Autodesk Inventor part; units mm, degrees
ref_plane "YZ Plane" through (0, 0, 0) normal (1, 0, 0) x (0, 1, 0)
ref_plane "XZ Plane" through (0, 0, 0) normal (0, 1, 0) x (-1, 0, 0)
ref_plane "XY Plane" through (0, 0, 0) normal (0, 0, 1) x (1, 0, 0)
sketch "Sketch1" plane through (0, 0, 0) normal (0, 0, 1) x (1, 0, 0)
  line L0 (0, 4) -> (0, 0)
  line L1 (0, 0) -> (125, 0)
  line L2 (125, 0) -> (125, 23.5)
  line L3 (57, 23.5) -> (0, 4)
  line L4 (81, 23.5) -> (81, 14.5)
  line L5 (81, 14.5) -> (92, 14.5)
  line L6 (92, 14.5) -> (92, 23.5)
  line L7 (125, 23.5) -> (92, 23.5)
  line L8 (81, 23.5) -> (57, 23.5)
  circle A0 centre (99.5, 19) radius 2.25
  circle A1 centre (119.5, 19) radius 2.25
  circle A2 centre (28.2, 6) radius 2.25
  circle A3 centre (28.2, 6) radius 4.5 construction
  point P0 (92, 19)
  dimension "d0" = 4
  dimension "d1" = 125
  dimension "d2" = 9
  dimension "d3" = 11
  dimension "d4" = 33
  dimension "d5" = 24
  dimension "d6" = 23.5
  dimension "d7" = 4.5
  dimension "d8" = 4.5
  dimension "d9" = 5.5
  dimension "d10" = 20
  dimension "d11" = 4.5
  dimension "d12" = 9
  dimension "d13" = 6
  dimension "d14" = 28.2
extrude "Extrusion1" add sketch "Sketch1" along normal blind 6.5
sketch "Sketch2" plane through (0, 0, 6.5) normal (0, 0, 1) x (1, 0, 0)
  line L0 (0, 0) -> (125, 0)
  line L1 (125, 23.5) -> (92, 23.5)
  line L2 (17, 0) -> (25, 0)
  line L3 (25, 0) -> (25, -4.5)
  line L4 (23, -6.5) -> (19, -6.5)
  line L5 (17, -4.5) -> (17, 0)
  line L6 (96, 0) -> (104, 0)
  line L7 (104, 0) -> (104, -19)
  line L8 (102, -21) -> (98, -21)
  line L9 (96, -19) -> (96, 0)
  line L10 (68, 0) -> (76, 0)
  line L11 (76, 0) -> (76, -19)
  line L12 (74, -21) -> (70, -21)
  line L13 (68, -19) -> (68, 0)
  line L14 (92, 23.5) -> (100, 23.5)
  line L15 (100, 23.5) -> (100, 28)
  line L16 (98, 30) -> (94, 30)
  line L17 (92, 28) -> (92, 23.5)
  arc A0 (17, -4.5) -> (19, -6.5) centre (19, -4.5) ccw
  arc A1 (23, -6.5) -> (25, -4.5) centre (23, -4.5) ccw
  arc A2 (96, -19) -> (98, -21) centre (98, -19) ccw
  arc A3 (102, -21) -> (104, -19) centre (102, -19) ccw
  arc A4 (68, -19) -> (70, -21) centre (70, -19) ccw
  arc A5 (74, -21) -> (76, -19) centre (74, -19) ccw
  arc A6 (94, 30) -> (92, 28) centre (94, 28) ccw
  arc A7 (100, 28) -> (98, 30) centre (98, 28) ccw
  line L18 (92, 23.5) -> (92, 14.5)
  dimension "d17" = 2
  dimension "d18" = 17
  dimension "d20" = 8
  dimension "d21" = 8
  dimension "d22" = 8
  dimension "d24" = 6.5
  dimension "d25" = 43
  dimension "d26" = 20
  dimension "d29" = 8
  dimension "d40" = 6.5
  dimension "d41" = 2
  dimension "d42" = 2
  dimension "d45" = 21
sketch "Sketch3" plane through (0, 0, 6.5) normal (0, 0, 1) x (1, 0, 0)
  circle A0 centre (119.5, 19) radius 2.25
  circle A1 centre (109.5, 19.599) radius 2.75
  circle A2 centre (86.5, 19.599) radius 7.5 construction
  dimension "d35" = 5.5
  dimension "d36" = 15
  dimension "d37" = 10
extrude "Extrusion3" cut sketch "Sketch3" against normal blind 6.5 contours A1
extrude "Extrusion4" add sketch "Sketch2" against normal blind 6.5
properties part number "x_motor_upper_nut_stop"
Check sheet for the modelled part. Datum: model origin and axes. Units: mm. A direction names the side the tool comes from. Round coordinates to 2 decimals unless told otherwise and drop trailing zeros. Loops run counter-clockwise (first coordinate to the right, second up) from the corner with the lowest first, then second, coordinate; pieces in that order, holes last.
1. Sectioned sample at B-B on x = 119.5. Record the boundary of the cut face in (y, z), and give its area (4 significant figures).
2. Set-up check for faces 1 (the flat face through (114, 0, 3)), 2 (the flat face through (113, 23.5, 3)), 3 (the flat face through (25, -2, 3)), 4 (the flat face through (8, 0, 3)), 5 (the flat face through (69, 23.5, 3)): record each of +Z, -Z, +X, -X, +Y, -Y from which the full face is reachable in a straight line by a thin tool's end or side.
3. Sectioned sample at A-A on y = -15.5. Record the boundary of the cut face in (x, z).
4. Scan lines: probe 1 along X at (y, z) = (-1, 5); probe 2 along X at (y, z) = (-6, 3.5); probe 3 along X at (y, z) = (-9, 4.5). Record each from-to range of solid material in increasing order.
5. Sectioned sample at D-D on z = 3. Give the number of separate pieces and of enclosed holes in the cut face, and give its area (3 significant figures).
6. Mould release check, pull along Y, two halves, no side actions. Record for faces 6 (the flat face through (28.899, 13.887, 3.204)), 7 (the cylindrical face through (29.41, 4.103, 3.204)), 8 (the flat face through (125, 12, 3)): released by +Y, released by -Y, zero draft, split by the parting line, or undercut.
7. Gauge pin test, flat ends, axial feed: pin 1 Ø3 at (x, z) = (73.5, 4) entering from +Y; pin 2 Ø1.2 at (x, z) = (21.5, 4.5) entering from -Y; pin 3 Ø3 at (x, z) = (40, 3.5) entering from -Y. Record the tip position at first contact, or that the pin passes through.
8. Sectioned sample at C-C on x = 83. Record the boundary of the cut face in (y, z), and give its area (4 significant figures).
Recorded:
1. outline: (0, 0) - (16.75, 0) - (16.75, 6.5) - (0, 6.5) - close; (21.25, 0) - (23.5, 0) - (23.5, 6.5) - (21.25, 6.5) - close
1. area: 123.5 mm2
2. face 1: +Z, -Z, +X, -Y
2. face 2: +Z, -Z, +X, +Y
2. face 3: +Z, -Z, -Y
2. face 4: +Z, -Z, -X, -Y
2. face 5: +Z, -Z, -X, +Y
3. outline: (68, 0) - (76, 0) - (76, 6.5) - (68, 6.5) - close; (96, 0) - (104, 0) - (104, 6.5) - (96, 6.5) - close
4. probe 1: x = 17 to 25, 68 to 76, 96 to 104
4. probe 2: x = 17.68 to 24.32, 68 to 76, 96 to 104
4. probe 3: x = 68 to 76, 96 to 104
5. separate pieces: 1
5. enclosed holes: 4
5. area: 2,640 mm2
6. face 6: released by +Y
6. face 7: undercut
6. face 8: zero draft
7. pin 1: stops at y = 23.5
7. pin 2: stops at y = -6.5
7. pin 3: stops at y = 0
8. outline: (0, 0) - (14.5, 0) - (14.5, 6.5) - (0, 6.5) - close
8. area: 94.25 mm2
